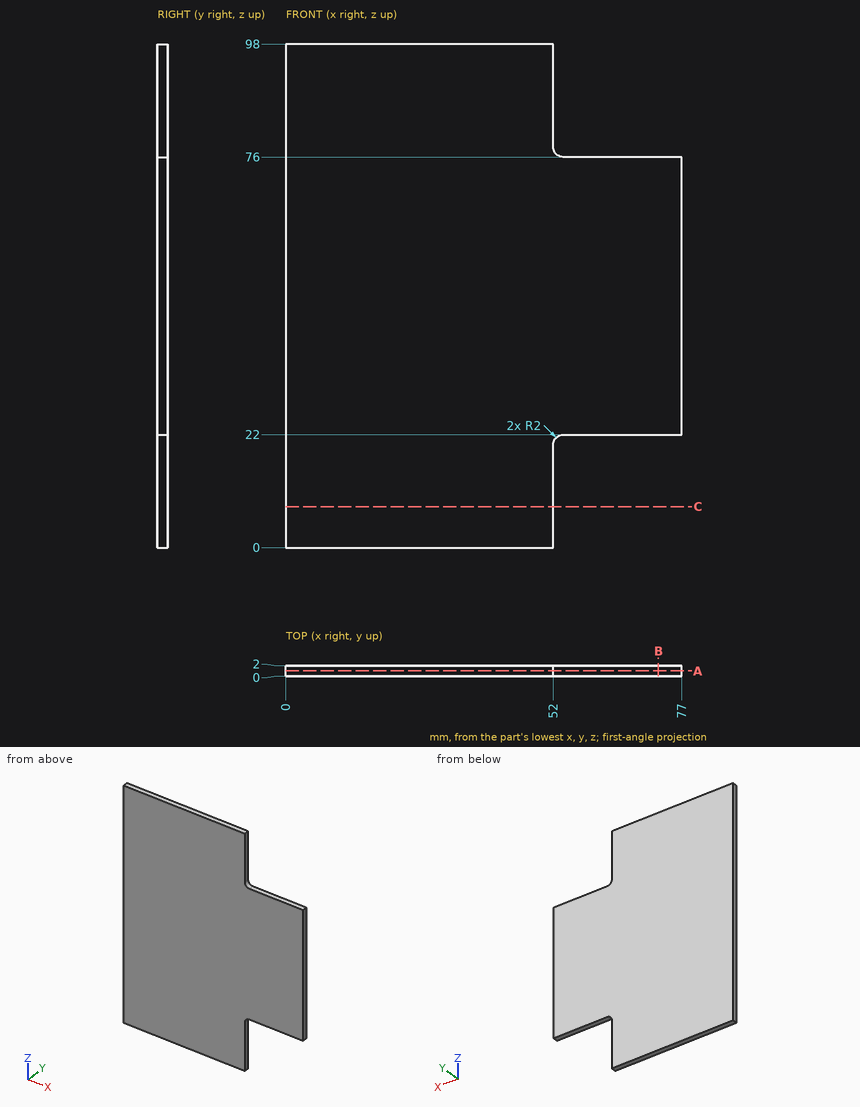
Job drawing, mm, ordinate dimensions from the low corner. One solid piece. Give positions to 0.01 mm unless a question says otherwise; leave off trailing zeros. Order: outer loops, then holes, each group sorted by start corner. A loop starts at its lowest first (then second) coordinate and runs counter-clockwise, first axis right, second up. Notation, with made-up numbers: M -31,69.25 L 2,69.25 A30 cw 2,101.25 Z; hole C -21.75,77 d3. An arc over 180 degrees is marked long. Put each result on its own line as item: value. Start each with the question number.
(1) Band-saw the part on B-B on x = 72.5. Give the cut face in (y, z), then the cut area to 3 significant figures.
(2) Pin check, flat tips, straight feed: pin 1 Ø0.6 at (y, z) = (1.5, 90) entering from +X; pin 2 Ø0.6 at (x, y) = (61, 1) entering from -Z; pin 3 Ø0.6 at (x, y) = (63, 1) entering from +Z. Stop position of each tip, or through.
(3) Band-saw the part on C-C on z = 8. Give the cut face in (x, y).
(4) Drill centre lines: L1, parallel to X at y = 0.15, z = 18.5; L2, parallel to Z at x = 55.5, y = 1.75. Where is each one in solid material? Low to high. Write a range as [from, to].
(5) Band-saw the part on A-A on y = 1. Give the cut face in (x, z), then the cut area to 3 significant figures.
Results below:
1. outline: M 0,22 L 2,22 L 2,76 L 0,76 Z
1. area: 108 mm2
2. pin 1: stops at x = 52
2. pin 2: stops at z = 22
2. pin 3: stops at z = 76
3. outline: M 0,0 L 52,0 L 52,2 L 0,2 Z
4. L1: x = [0, 52]
4. L2: z = [22, 76]
5. outline: M 0,0 L 52,0 L 52,20 A2 cw 54,22 L 77,22 L 77,76 L 54,76 A2 cw 52,78 L 52,98 L 0,98 Z
5. area: 6,450 mm2
